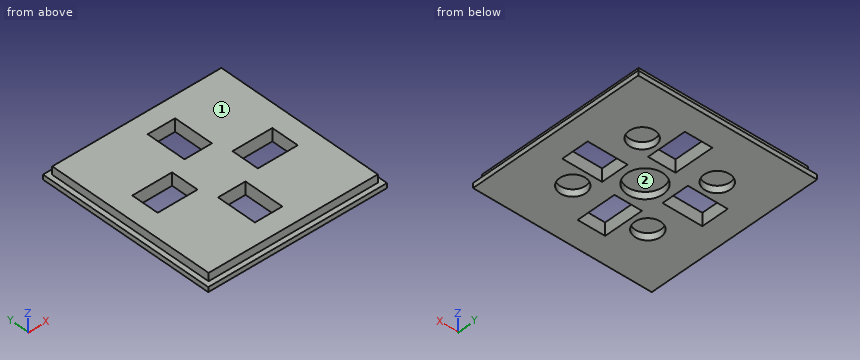
Autodesk Inventor part; units mm, degrees
ref_plane "YZ Plane" through (0, 0, 0) normal (1, 0, 0) x (0, 1, 0)
ref_plane "XZ Plane" through (0, 0, 0) normal (0, 1, 0) x (-1, 0, 0)
sketch "Skizze1" plane through (0, 0, 0) normal (0, 0, 1) x (1, 0, 0)
  line L0 (-28.13, 28.13) -> (28.13, 28.13)
  line L1 (28.13, 28.13) -> (28.13, -28.13)
  line L2 (28.13, -28.13) -> (-28.13, -28.13)
  line L3 (-28.13, -28.13) -> (-28.13, 28.13)
  line L4 (-39.382, 0) -> (39.382, 0) construction
  line L5 (0, -39.382) -> (0, 39.382) construction
  point P0 (0, 0)
  dimension "d0" = 56.26
extrude "Extrusion1" add sketch "Skizze1" along normal blind 1.5
sketch "Skizze2" plane through (0, 0, 1.5) normal (0, 0, 1) x (1, 0, 0)
  line L0 (0, -39.382) -> (0, 39.382) construction
  line L1 (-39.382, 0) -> (39.382, 0) construction
  line L2 (-26.6175, 26.6175) -> (26.6175, 26.6175)
  line L3 (26.6175, 26.6175) -> (26.6175, -26.6175)
  line L4 (26.6175, -26.6175) -> (-26.6175, -26.6175)
  line L5 (-26.6175, -26.6175) -> (-26.6175, 26.6175)
  line L6 (28.13, 28.13) -> (-28.13, 28.13)
  point P0 (0, 0)
  dimension "d3" = 53.235
extrude "Extrusion2" add sketch "Skizze2" along normal blind 2.5
sketch "Skizze3" plane through (0, 0, 0) normal (0, 0, -1) x (-1, 0, 0)
  line L0 (28.13, -28.13) -> (-28.13, -28.13)
  line L1 (28.13, 28.13) -> (28.13, -28.13)
  line L2 (-28.13, 28.13) -> (28.13, 28.13)
  line L3 (-28.13, -28.13) -> (-28.13, 28.13)
  line L4 (-6.21, 20.295) -> (2.43, 20.295)
  line L5 (2.43, 20.295) -> (2.43, 7.76)
  line L6 (2.43, 7.76) -> (-6.21, 7.76)
  line L7 (-6.21, 7.76) -> (-6.21, 20.295)
  point P0 (0, 0)
  point P1 (0, 0)
  dimension "d6" = 21.92
  dimension "d7" = 8.64
  dimension "d8" = 12.535
  dimension "d9" = 35.89
extrude "Extrusion3" cut sketch "Skizze3" against normal up to surface (4 mm away) contours L4 L5 L6 L7
pattern_circular "Runde Anordnung1" count 4 over 360 about axis through (0, 0, -10) along (0, 0, 1) of "Extrusion3"
sketch "Skizze4" plane through (0, 0, 0) normal (0, 0, -1) x (-1, 0, 0)
  line L0 (-28.13, -28.13) -> (-28.13, 28.13)
  line L1 (-28.13, 28.13) -> (28.13, 28.13)
  point P0 (0, 0)
  point P1 (-11.817, 11.817)
  dimension "d15" = 16.313
  dimension "d16" = 16.313
hole "Bohrung1" at (11.817, 11.817, 0) direction (0, 0, 1) diameter 5.5 depth 3.55 counterbore diameter 8.2 counterbore depth 2.2
pattern_circular "Runde Anordnung2" count 4 over 360 about axis through (0, 0, -10) along (0, 0, 1) of "Bohrung1"
sketch "Skizze5" plane through (0, 0, 0) normal (0, 0, -1) x (-1, 0, 0)
  point P0 (0, 0)
  point P1 (0, 0)
hole "Bohrung2" at (0, 0, 0) direction (0, 0, 1) diameter 5.5 depth 3.55 counterbore diameter 11.4 counterbore depth 2.2
ref_plane "Arbeitsebene1" through (0, 0, 2.2) normal (0, 0, 1) x (1, 0, 0)
sketch "Skizze6" plane through (0, 0, 2.2) normal (0, 0, 1) x (1, 0, 0)
  circle A0 centre (-11.817, -11.817) radius 2.75
  circle A1 centre (-11.817, 11.817) radius 2.75
  circle A2 centre (11.817, 11.817) radius 2.75
  circle A3 centre (11.817, -11.817) radius 2.75
  circle A4 centre (0, 0) radius 2.75
extrude "Extrusion4" add sketch "Skizze6" along normal blind 0.2
properties part number "PCB_coverPlatte_MagnetEingefasst"
Can you work these out from the model? Positions are in its coordinate system, mm. Face numbers are marked on the shaded views. Coordinates: 2 decimals unless noted, no trailing zeros. Write each loop counter-clockwise with the first axis right and the second up, starting at its lowest first coordinate (ties: lowest second). Pieces come first, ordered by that corner, then holes. Notation, with made-up numbers: (-0.5, -37) - (3.5, -37) arc R27 ccw to (3.5, -15) - close; hole circle Ø4 at (25, 36). An arc over 180 degrees is marked (long way). Return JSON: item names as keys, results as strings.
Q1. If we section it at C-C (y = 18.5): Please give me the cut outline in (x, z), then the cut area to 3 significant figures.
Computed values:
{"outline": "(-28.13, 0) - (-2.43, 0) - (-2.43, 4) - (-26.62, 4) - (-26.62, 1.5) - (-28.13, 1.5) - close; (6.21, 0) - (28.13, 0) - (28.13, 1.5) - (26.62, 1.5) - (26.62, 4) - (6.21, 4) - close", "area": "183 mm2"}
Q2. Please list where these lines run through material, in increasing order: L1, parallel to X at y = -16, z = 3.8; L2, parallel to Y at x = -2.5, z = 0.3 (1 decimal); L3, parallel to Y at x = 2, z = 1.95 (1 decimal). Write a range as from..to.
Computed values:
{"L1": "x = -26.62..-6.21, 2.43..26.62", "L2": "y = -28.1..-20.3, -7.8..-5.1, 5.1..28.1", "L3": "y = -26.6..-20.3, -7.8..-5.3, 5.3..7.8, 20.3..26.6"}
Q3. Thinking about a two-plate mould opening in Y: for the marked faces 1 and 2, which applies, +Y half, -Y half, draft (parallel to the pull), parting line (faces both ways), or undercut?
Computed values:
{"face 1": "draft", "face 2": "undercut"}
Q4. If we section it at D-D (x = 17): Please give me the cut outline in (y, z).
Computed values:
{"outline": "(-28.13, 0) - (-6.21, 0) - (-6.21, 4) - (-26.62, 4) - (-26.62, 1.5) - (-28.13, 1.5) - close; (2.43, 0) - (28.13, 0) - (28.13, 1.5) - (26.62, 1.5) - (26.62, 4) - (2.43, 4) - close"}
Q5. If we section it at A-A (y = 0): Count the separate pieces of the cut face and the enclosed holes in it, then the cut area to 3 significant figures.
Computed values:
{"separate pieces": "3", "enclosed holes": "1", "area": "85.8 mm2"}
Q6. I'm going to push flat-ended pins straight in: pin 1 Ø4.5 at (x, y) = (11.817, 11.817) entering from -Z; pin 2 Ø1.2 at (x, z) = (14, 2.5) entering from -Y. Where does each tip first touch, or does it pass through?
Computed values:
{"pin 1": "stops at z = 2.2", "pin 2": "stops at y = -26.62"}
